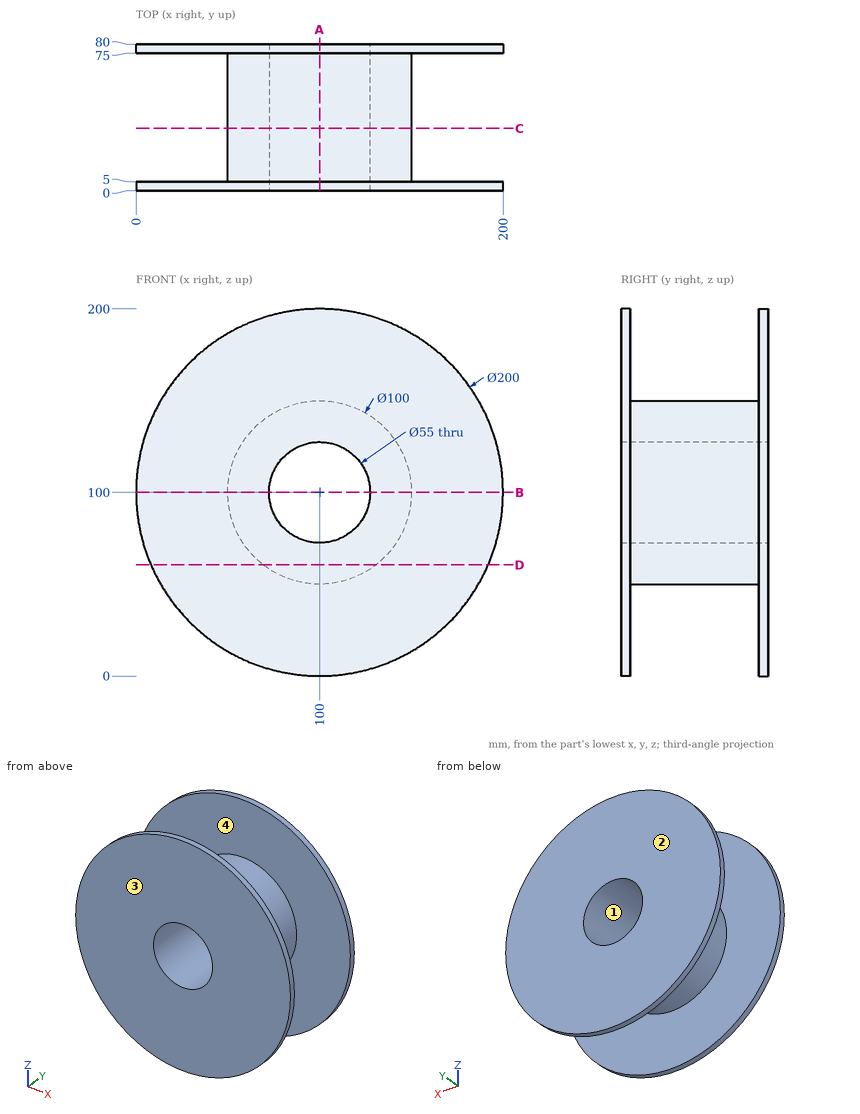
For this review, use the dimensioned drawing (mm, ordinates from the lowest corner) and the shaded views. Coordinates: 2 decimals unless noted, no trailing zeros. Loops run counter-clockwise (first coordinate to the right, second up) from the corner with the lowest first, then second, coordinate; pieces in that order, holes last. Notation, with made-up numbers: (26.5, 87) -> (41.5, 87) arc R23 cw to (41.5, 99) -> close; hole circle Ø3 at (59.5, 53). An arc over 180 degrees is marked (long way). Use a Markdown table: item, result. Add a question column.
Item 1: We need section D-D, the plane z = 60.5. Write out the cut boundary in (x, y), and give its area (3 significant figures).
Item 2: The part is to be moulded in two halves that separate along Y. For the marked faces 1, 2, 3 and 4, say which applies: +Y half, -Y half, draft (parallel to the pull), parting line (faces both ways), or undercut.
Item 3: We need section A-A, the plane x = 100. Write out the cut boundary in (y, z), and give its area (3 significant figures).
Item 4: We need section C-C, the plane y = 34. Write out the cut boundary in (x, z), and give its area (3 significant figures).
Item 5: Clearance check with flat-ended pins moving along their axes: P1, Ø10, axis at x = 119, z = 141.5, coming from the -Y side; P2, Ø8, axis at x = 149.5, y = 50, coming from the -Z side; P3, Ø4, axis at y = 47, z = 55, coming from the +X side; P4, Ø1, axis at x = 116.5, y = 49.5, coming from the +Z side. State where each tip first meets the part, or that it passes through.
Item 6: Wall thickness on L1, parallel to Y at x = 144, z = 33; L2, parallel to Z at x = 100, y = 45; L3, parallel to Z at x = 106, y = 76.5: over which ranges is each line inside the solid? List them lowest first. Write a range as from..to.
Item 7: We need section B-B, the plane z = 100. Write out the cut boundary in (x, y).
Numbers:
| question | item | result |
|---|---|---|
| 1 | outline | (8.13, 0) -> (191.87, 0) -> (191.87, 5) -> (130.66, 5) -> (130.66, 75) -> (191.87, 75) -> (191.87, 80) -> (8.13, 80) -> (8.13, 75) -> (69.34, 75) -> (69.34, 5) -> (8.13, 5) -> close |
| 1 | area | 6,130 mm^2 |
| 2 | face 1 | draft |
| 2 | face 2 | +Y half |
| 2 | face 3 | -Y half |
| 2 | face 4 | undercut |
| 3 | outline | (0, 0) -> (5, 0) -> (5, 50) -> (75, 50) -> (75, 0) -> (80, 0) -> (80, 72.5) -> (0, 72.5) -> close; (0, 127.5) -> (80, 127.5) -> (80, 200) -> (75, 200) -> (75, 150) -> (5, 150) -> (5, 200) -> (0, 200) -> close |
| 3 | area | 4,600 mm^2 |
| 4 | outline | circle Ø100 at (100, 100); hole circle Ø55 at (100, 100) |
| 4 | area | 5,480 mm^2 |
| 5 | P1 | stops at y = 0 |
| 5 | P2 | stops at z = 79.27 |
| 5 | P3 | stops at x = 125.51 |
| 5 | P4 | stops at z = 147.37 |
| 6 | L1 | y = 0..5, 75..80 |
| 6 | L2 | z = 50..72.5, 127.5..150 |
| 6 | L3 | z = 0.18..73.16, 126.84..199.82 |
| 7 | outline | (0, 0) -> (72.5, 0) -> (72.5, 80) -> (0, 80) -> (0, 75) -> (50, 75) -> (50, 5) -> (0, 5) -> close; (127.5, 0) -> (200, 0) -> (200, 5) -> (150, 5) -> (150, 75) -> (200, 75) -> (200, 80) -> (127.5, 80) -> close |
